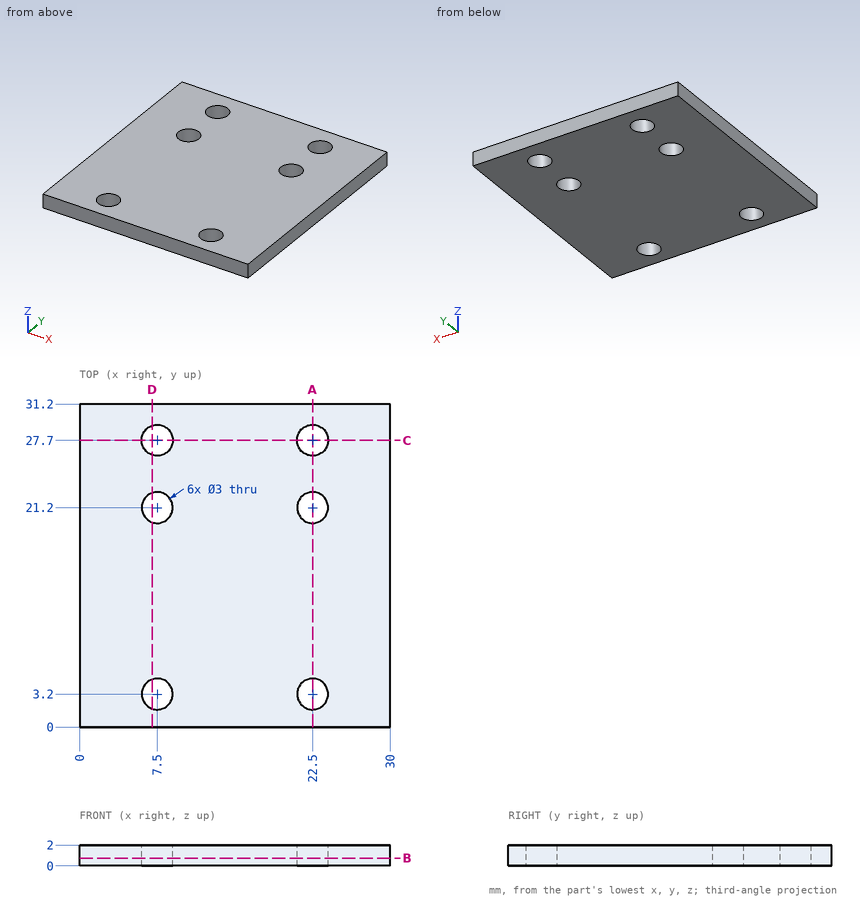
The figure shows three views and two pictorial views of one solid part (mm, origin at its lowest corner). Answer the questions. Give positions to 0.01 mm unless a question says otherwise; leave off trailing zeros. Order: outer loops, then holes, each group sorted by start corner. A loop starts at its lowest first (then second) coordinate and runs counter-clockwise, first axis right, second up. Notation, with made-up numbers: (26.25, 6.25) -> (70.25, 6.25) arc R9 ccw to (70.25, 12.25) -> close; hole circle Ø9 at (14, 61.25). An arc over 180 degrees is marked (long way). Answer as CSV lines item,"result". Start each with the question number.
Q1. Find the intervals of material crossed by L1, parallel to Y at x = 7.5, z = 0.45; L2, parallel to X at y = 20, z = 0.75; L3, parallel to X at y = 3.5, z = 0.5, in increasing order.
Q2. A cutting plane is placed at B-B (z = 0.75). Determine the outline of the cut face in (x, y).
Q3. A cutting plane is placed at D-D (x = 7). Determine the outline of the cut face in (y, z).
Q4. Given pin 1 (4 mm diameter, centred on x = 7.5, y = 27.7, fed in from -Z); pin 2 (1.8 mm diameter, centred on x = 7.5, y = 21.2, fed in from +Z), each flat-ended and moving along its own axis, determine where each tip first touches the part or whether it passes through.
Q5. A cutting plane is placed at A-A (x = 22.5). Determine the outline of the cut face in (y, z).
Q6. A cutting plane is placed at C-C (y = 27.7). Determine the outline of the cut face in (x, z).
Results found:
1,L1,"0 to 1.7, 4.7 to 19.7, 22.7 to 26.2, 29.2 to 31.2"
1,L2,"0 to 6.6, 8.4 to 21.6, 23.4 to 30"
1,L3,"0 to 6.03, 8.97 to 21.03, 23.97 to 30"
2,outline,"(0, 0) -> (30, 0) -> (30, 31.2) -> (0, 31.2) -> close; hole circle Ø3 at (7.5, 3.2); hole circle Ø3 at (7.5, 21.2); hole circle Ø3 at (7.5, 27.7); hole circle Ø3 at (22.5, 3.2); hole circle Ø3 at (22.5, 21.2); hole circle Ø3 at (22.5, 27.7)"
3,outline,"(0, 0) -> (1.79, 0) -> (1.79, 2) -> (0, 2) -> close; (4.61, 0) -> (19.79, 0) -> (19.79, 2) -> (4.61, 2) -> close; (22.61, 0) -> (26.29, 0) -> (26.29, 2) -> (22.61, 2) -> close; (29.11, 0) -> (31.2, 0) -> (31.2, 2) -> (29.11, 2) -> close"
4,pin 1,"z = 0"
4,pin 2,"through"
5,outline,"(0, 0) -> (1.7, 0) -> (1.7, 2) -> (0, 2) -> close; (4.7, 0) -> (19.7, 0) -> (19.7, 2) -> (4.7, 2) -> close; (22.7, 0) -> (26.2, 0) -> (26.2, 2) -> (22.7, 2) -> close; (29.2, 0) -> (31.2, 0) -> (31.2, 2) -> (29.2, 2) -> close"
6,outline,"(0, 0) -> (6, 0) -> (6, 2) -> (0, 2) -> close; (9, 0) -> (21, 0) -> (21, 2) -> (9, 2) -> close; (24, 0) -> (30, 0) -> (30, 2) -> (24, 2) -> close"
